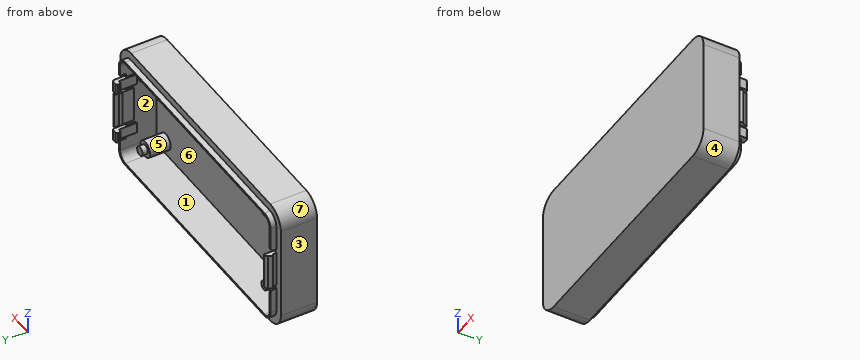
from build123d import *

# Parameters (mm, degrees)
EXTRUDE_2_DEPTH       = 10
EXTRUDE_4_DEPTH       = 1.6
SKETCH_7_W            = 0.5
SKETCH_7_H            = 10
EXTRUDE_8_DEPTH       = 2.8
SKETCH_8_R            = 0.7
EXTRUDE_9_DEPTH       = 10
FILLET_1_R            = 0.5
SKETCH_11_W           = 1
SKETCH_11_H           = 1.6
CUT_EXTRUDE_1_DEPTH   = 1.2
FILLET_2_R            = 1
SKETCH_13_W           = 0.5
SKETCH_13_H           = 10
EXTRUDE_10_DEPTH      = 2.8
CUT_EXTRUDE_START     = -8.5
CUT_EXTRUDE_2_DEPTH   = 8.5
SKETCH_13_2_W         = 0.5
SKETCH_13_2_H         = 10
EXTRUDE_11_DEPTH      = 2
EXTRUDE_12_DEPTH      = 1.6
EXTRUDE_12_DEPTH_BACK = 2
SKETCH_5_W            = 0.3
SKETCH_5_H            = 10
SKETCH_15_R           = 2.25
EXTRUDE_13_DEPTH      = 5.7
SKETCH_16_R           = 1.25
EXTRUDE_14_DEPTH      = 1.5
SKETCH_17_W           = 0.5
SKETCH_17_H           = 1
CUT_EXTRUDE_3_DEPTH   = 1.6
SKETCH_19_W           = 0.8
SKETCH_19_H           = 10
EXTRUDE_15_DEPTH      = 1.8
SKETCH_20_R           = 0.7
EXTRUDE_16_DEPTH      = 10
FILLET_4_R            = 0.5
SKETCH_21_W           = 0.5
SKETCH_21_H           = 3
EXTRUDE_17_DEPTH      = 1.9
SKETCH_22_W           = 3
SKETCH_22_H           = 6.3
EXTRUDE_23_DEPTH      = 0.5
FILLET_12_R           = 0.5
SKETCH_29_W           = 0.5
SKETCH_29_H           = 1
CUT_EXTRUDE_5_DEPTH   = 1.6
SKETCH_30_W           = 3
SKETCH_30_H           = 1.3
EXTRUDE_26_DEPTH      = 1
CHAMFER_7_SIZE        = 0.4


with BuildPart() as part:
    # case 2 → 凸台-拉伸2 (new body)
    with BuildSketch(Plane(origin=(0, 0, 0), x_dir=(1, 0, 0), z_dir=(0, 1, 0))):
        with BuildLine():
            Line((-34.042196447, 18), (30.957803553, 18))
            ThreePointArc((30.957803553, 18), (34.493337459, 16.535533906), (35.957803553, 13))
            Line((35.957803553, 13), (35.957803553, -13))
            ThreePointArc((35.957803553, -13), (34.493337459, -16.535533906), (30.957803553, -18))
            Line((30.957803553, -18), (-34.042196447, -18))
            ThreePointArc((-34.042196447, -18), (-37.577730353, -16.535533906), (-39.042196447, -13))
            Line((-39.042196447, -13), (-39.042196447, 13))
            ThreePointArc((-39.042196447, 13), (-37.577730353, 16.535533906), (-34.042196447, 18))
        make_face()
    extrude(amount=EXTRUDE_2_DEPTH)

    # 草图3 → 凸台-拉伸4 (add)
    with BuildSketch(Plane(origin=(0, 10, 0), x_dir=(1, 0, 0), z_dir=(0, 1, 0))):
        with BuildLine():
            Line((-36.942196447, 13), (-36.942196447, -13))
            ThreePointArc((-36.942196447, -13), (-36.092806113, -15.050609665), (-34.042196447, -15.9))
            Line((-34.042196447, -15.9), (30.957803553, -15.9))
            ThreePointArc((30.957803553, -15.9), (33.008413218, -15.050609665), (33.857803553, -13))
            Line((33.857803553, -13), (33.857803553, 13))
            ThreePointArc((33.857803553, 13), (33.008413218, 15.050609665), (30.957803553, 15.9))
            Line((30.957803553, 15.9), (-34.042196447, 15.9))
            ThreePointArc((-34.042196447, 15.9), (-36.092806113, 15.050609665), (-36.942196447, 13))
        make_face()
        with BuildLine():
            Line((-34.042196447, -15.4), (30.957803553, -15.4))
            ThreePointArc((30.957803553, -15.4), (32.654859828, -14.697056275), (33.357803553, -13))
            Line((33.357803553, -13), (33.357803553, 13))
            ThreePointArc((33.357803553, 13), (32.654859828, 14.697056275), (30.957803553, 15.4))
            Line((30.957803553, 15.4), (-34.042196447, 15.4))
            ThreePointArc((-34.042196447, 15.4), (-35.739252722, 14.697056275), (-36.442196447, 13))
            Line((-36.442196447, 13), (-36.442196447, -13))
            ThreePointArc((-36.442196447, -13), (-35.739252722, -14.697056275), (-34.042196447, -15.4))
        make_face(mode=Mode.SUBTRACT)
    extrude(amount=EXTRUDE_4_DEPTH)

    # 草图7 → 凸台-拉伸8 (add)
    with BuildSketch(Plane(origin=(0, 10, 0), x_dir=(1, 0, 0), z_dir=(0, 1, 0))):
        with Locations((-36.692196447, 0)):
            Rectangle(SKETCH_7_W, SKETCH_7_H)
    extrude(amount=EXTRUDE_8_DEPTH)

    # 草图8 → 凸台-拉伸9 (add)
    with BuildSketch(Plane.XY.offset(5)):
        with Locations((-36.692196447, 11.6)):
            Circle(SKETCH_8_R)
    extrude(amount=-EXTRUDE_9_DEPTH)

    # 圆角1
    fillet_1_edges = [part.edges().sort_by_distance(p)[0] for p in [
        (-36.942196447, 12.8, 0),
    ]]
    fillet(fillet_1_edges, radius=FILLET_1_R - 0.0001)  # a hair under: the kernel refuses the full size

    # 草图11 → 切除-拉伸1 (cut)
    with BuildSketch(Plane.ZY.offset(36.942196447)):
        with Locations((5.5, 10.8)):
            Rectangle(SKETCH_11_W, SKETCH_11_H)
        with Locations((-5.5, 10.8)):
            Rectangle(SKETCH_11_W, SKETCH_11_H)
    extrude(amount=-CUT_EXTRUDE_1_DEPTH, mode=Mode.SUBTRACT)

    # 圆角2
    fillet_2_edges = [part.edges().sort_by_distance(p)[0] for p in [
        (-36.692196447, 11.6, 6),
        (-36.692196447, 11.6, -6),
    ]]
    fillet(fillet_2_edges, radius=FILLET_2_R)

    # 草图13 → 凸台-拉伸10 (add)
    with BuildSketch(Plane(origin=(0, 10, 0), x_dir=(1, 0, 0), z_dir=(0, 1, 0))):
        with Locations((-36.192196447, 0)):
            Rectangle(SKETCH_13_W, SKETCH_13_H)
    extrude(amount=EXTRUDE_10_DEPTH)

    # 草图14 → 切除-拉伸2 (cut)
    with BuildSketch(Plane(origin=(0, 10, 0), x_dir=(1, 0, 0), z_dir=(0, 1, 0)).offset(CUT_EXTRUDE_START)):
        with BuildLine():
            Line((-34.042196447, -15.4), (30.957803553, -15.4))
            ThreePointArc((30.957803553, -15.4), (32.654859828, -14.697056275), (33.357803553, -13))
            Line((33.357803553, -13), (33.357803553, 13))
            ThreePointArc((33.357803553, 13), (32.654859828, 14.697056275), (30.957803553, 15.4))
            Line((30.957803553, 15.4), (-34.042196447, 15.4))
            ThreePointArc((-34.042196447, 15.4), (-35.739252722, 14.697056275), (-36.442196447, 13))
            Line((-36.442196447, 13), (-36.442196447, -13))
            ThreePointArc((-36.442196447, -13), (-35.739252722, -14.697056275), (-34.042196447, -15.4))
        make_face()
    extrude(amount=CUT_EXTRUDE_2_DEPTH, mode=Mode.SUBTRACT)

    # 草图13<2> → 凸台-拉伸11 (add)
    with BuildSketch(Plane(origin=(0, 10, 0), x_dir=(1, 0, 0), z_dir=(0, 1, 0))):
        with Locations((-36.192196447, 0)):
            Rectangle(SKETCH_13_2_W, SKETCH_13_2_H)
    extrude(amount=-EXTRUDE_11_DEPTH)

    # 草图5 → 凸台-拉伸12 (add, two sides: drawn at the far end of the back side and taken through both)
    with BuildSketch(Plane(origin=(0, 10, 0), x_dir=(1, 0, 0), z_dir=(0, 1, 0)).offset(-EXTRUDE_12_DEPTH_BACK)):
        with Locations((33.207803553, 0)):
            Rectangle(SKETCH_5_W, SKETCH_5_H)
    extrude(amount=EXTRUDE_12_DEPTH + EXTRUDE_12_DEPTH_BACK)

    # 草图15 → 凸台-拉伸13 (add)
    with BuildSketch(Plane(origin=(0, 1.5, 0), x_dir=(1, 0, 0), z_dir=(0, 1, 0))):
        with Locations(Location((29.060337171, -11.529492838, 0), (0, 0, 270))):
            Circle(SKETCH_15_R)
        with Locations(Location((-28.939662829, -11.529492838, 0), (0, 0, 270))):
            Circle(SKETCH_15_R)
        with Locations(Location((29.060337171, 11.470507162, 0), (0, 0, 270))):
            Circle(SKETCH_15_R)
        with Locations(Location((-28.939662829, 11.470507162, 0), (0, 0, 270))):
            Circle(SKETCH_15_R)
    extrude(amount=EXTRUDE_13_DEPTH)

    # 草图16 → 凸台-拉伸14 (add)
    with BuildSketch(Plane(origin=(0, 7.2, 0), x_dir=(1, 0, 0), z_dir=(0, 1, 0))):
        with Locations(Location((29.060337171, -11.529492838, 0), (0, 0, 270))):
            Circle(SKETCH_16_R)
        with Locations(Location((29.060337171, 11.470507162, 0), (0, 0, 270))):
            Circle(SKETCH_16_R)
        with Locations(Location((-28.939662829, -11.529492838, 0), (0, 0, 270))):
            Circle(SKETCH_16_R)
        with Locations(Location((-28.939662829, 11.470507162, 0), (0, 0, 270))):
            Circle(SKETCH_16_R)
    extrude(amount=EXTRUDE_14_DEPTH)

    # 草图17 → 切除-拉伸3 (cut)
    with BuildSketch(Plane(origin=(0, 11.6, 0), x_dir=(1, 0, 0), z_dir=(0, 1, 0))):
        with Locations((33.607803553, -5.5)):
            Rectangle(SKETCH_17_W, SKETCH_17_H)
        with Locations((33.607803553, 5.5)):
            Rectangle(SKETCH_17_W, SKETCH_17_H)
    extrude(amount=-CUT_EXTRUDE_3_DEPTH, mode=Mode.SUBTRACT)

    # 草图19 → 凸台-拉伸15 (add)
    with BuildSketch(Plane(origin=(0, 11.6, 0), x_dir=(1, 0, 0), z_dir=(0, 1, 0))):
        with Locations((33.457803553, 0)):
            Rectangle(SKETCH_19_W, SKETCH_19_H)
    extrude(amount=EXTRUDE_15_DEPTH)

    # 草图20 → 凸台-拉伸16 (add)
    with BuildSketch(Plane(origin=(0, 0, -5), x_dir=(-1, 0, 0), z_dir=(0, 0, -1))):
        with Locations((-33.607803553, 11.6)):
            Circle(SKETCH_20_R)
    extrude(amount=-EXTRUDE_16_DEPTH)

    # 圆角4
    fillet_4_edges = [part.edges().sort_by_distance(p)[0] for p in [
        (33.857803553, 13.4, 0),
    ]]
    fillet(fillet_4_edges, radius=FILLET_4_R)

    # 草图21 → 凸台-拉伸17 (add)
    with BuildSketch(Plane(origin=(0, 11.6, 0), x_dir=(1, 0, 0), z_dir=(0, 1, 0))):
        with Locations((33.607803553, -7.5)):
            Rectangle(SKETCH_21_W, SKETCH_21_H)
        with Locations((33.607803553, 7.5)):
            Rectangle(SKETCH_21_W, SKETCH_21_H)
    extrude(amount=EXTRUDE_17_DEPTH)

    # 草图22 → 凸台-拉伸23 (add)
    with BuildSketch(Plane.ZY.offset(-33.357803553)):
        with Locations((-7.5, 10.35)):
            Rectangle(SKETCH_22_W, SKETCH_22_H)
        with Locations((7.5, 10.35)):
            Rectangle(SKETCH_22_W, SKETCH_22_H)
    extrude(amount=EXTRUDE_23_DEPTH)

    # 圆角12
    fillet_12_edges = [part.edges().sort_by_distance(p)[0] for p in [
        (33.857803553, 13.5, 7.5),
        (33.857803553, 13.5, -7.5),
    ]]
    fillet(fillet_12_edges, radius=FILLET_12_R)

    # 草图29 → 切除-拉伸5 (cut)
    with BuildSketch(Plane(origin=(0, 11.6, 0), x_dir=(1, 0, 0), z_dir=(0, 1, 0))):
        with Locations((33.607803553, -9.5)):
            Rectangle(SKETCH_29_W, SKETCH_29_H)
        with Locations((33.607803553, 9.5)):
            Rectangle(SKETCH_29_W, SKETCH_29_H)
    extrude(amount=-CUT_EXTRUDE_5_DEPTH, mode=Mode.SUBTRACT)

    # 草图30 → 凸台-拉伸26 (add)
    with BuildSketch(Plane.ZY.offset(-32.857803553)):
        with Locations((7.5, 12.85)):
            Rectangle(SKETCH_30_W, SKETCH_30_H)
        with Locations((-7.5, 12.85)):
            Rectangle(SKETCH_30_W, SKETCH_30_H)
    extrude(amount=EXTRUDE_26_DEPTH)

    # 倒角7
    chamfer_7_edges = [part.edges().sort_by_distance(p)[0] for p in [
        (31.857803553, 12.2, 7.5),
        (31.857803553, 13.5, 7.5),
        (31.857803553, 12.2, -7.5),
        (31.857803553, 13.5, -7.5),
    ]]
    chamfer(chamfer_7_edges, length=CHAMFER_7_SIZE)


solid = part.part
For this review, take the finished solid that the model builds, in its own axes (mm). Face numbers are marked on the shaded views. A direction names the side the tool comes from. Round coordinates to 2 decimals unless told otherwise and drop trailing zeros. Write each loop counter-clockwise with the first axis right and the second up, starting at its lowest first coordinate (ties: lowest second). Pieces come first, ordered by that corner, then holes. Notation, with made-up numbers: M -25.5,37 L -20.5,37 A33 ccw -20.5,69 Z; hole C -37,78.25 d7. An arc over 180 degrees is marked long. Write item = value, one per line. Start each with the question number.
(1) We need section B-B (z = 0). Give the boundary of the cut face in (x, y), then the cut area to 3 significant figures.
(2) We need section D-D (z = 11). Give the boundary of the cut face in (x, y).
(3) For the marked faces 1, 2 and 3, list the 3-axis set-ups (+Z, -Z, +X, -X, +Y, -Y) from which the entire face can be reached by the end or side of a thin tool; tool diameter is ignored.
(4) We need section A-A (y = 3.75). Give the boundary of the cut face in (x, z), then the cut area to 3 significant figures.
(5) Clearance check with flat-ended pins moving along their axes: pin 1 Ø0.6 at (y, z) = (13, 7) entering from -X; pin 2 Ø0.8 at (x, z) = (-29, -11.5) entering from +Y; pin 3 Ø10 at (x, z) = (10.5, -10.5) entering from -Y; pin 4 Ø3.5 at (y, z) = (12, 7.5) entering from +X. State where each tip first meets the part, or that it passes through.
(6) For line 1 along X through (y, z) = (11.25, -7); line 2 along Z through (x, y) = (14, 10.5); line 3 along X through (y, z) = (10.25, -2.5), list the stretches that pass through material, from the lowest coordinate up.
(7) We need section C-C (x = -25). Give the boundary of the cut face in (y, z), then the cut area to 3 significant figures.
(8) The part is to be moulded in two halves that separate along Z. For the marked faces 4, 5, 6 and 7, say which applies: +Z half, -Z half, draft (parallel to the pull), parting line (faces both ways), or undercut.
Results found:
q1.outline = M -39.04,0 L 35.96,0 L 35.96,10 L 33.86,10 L 33.86,10.95 A0.7 ccw 33.86,12.25 L 33.86,12.9 A0.5 ccw 33.36,13.4 L 33.06,13.4 L 33.06,12.03 A0.7 ccw 33.06,11.17 L 33.06,8 L 33.36,8 L 33.36,1.5 L -36.44,1.5 L -36.44,8 L -35.94,8 L -35.94,12.8 L -36.44,12.8 A0.5 ccw -36.94,12.3 L -36.94,12.25 A0.7 ccw -36.94,10.95 L -36.94,10 L -39.04,10 Z
q1.area = 165 mm²
q2.outline = M -39.04,0 L 35.96,0 L 35.96,10 L 33.86,10 L 33.86,11.6 L 33.36,11.6 L 33.36,1.5 L 31.25,1.5 L 31.25,7.2 L 30.19,7.2 L 30.19,8.7 L 27.93,8.7 L 27.93,7.2 L 26.87,7.2 L 26.87,1.5 L -26.75,1.5 L -26.75,7.2 L -27.81,7.2 L -27.81,8.7 L -30.07,8.7 L -30.07,7.2 L -31.13,7.2 L -31.13,1.5 L -36.44,1.5 L -36.44,11.6 L -36.94,11.6 L -36.94,10 L -39.04,10 Z
q3.face_1 = +Y
q3.face_2 = none
q3.face_3 = +Z, -Z, -X, +Y, -Y
q4.outline = M -39.04,-13 A5 ccw -34.04,-18 L 30.96,-18 A5 ccw 35.96,-13 L 35.96,13 A5 ccw 30.96,18 L -34.04,18 A5 ccw -39.04,13 Z; C -28.94,-11.47 d4.5; C -28.94,11.53 d4.5; C 29.06,-11.47 d4.5; C 29.06,11.53 d4.5; hole M -36.44,-13 A2.4 ccw -34.04,-15.4 L 30.96,-15.4 A2.4 ccw 33.36,-13 L 33.36,13 A2.4 ccw 30.96,15.4 L -34.04,15.4 A2.4 ccw -36.44,13 Z
q4.area = 597 mm²
q5.pin_1 = 31.86
q5.pin_2 = 8.7
q5.pin_3 = 0
q5.pin_4 = 33.86
q6.line_1 = -36.94 to -36.44, 32.86 to 33.86
q6.line_2 = -15.9 to -15.4, 15.4 to 15.9
q6.line_3 = -36.94 to -35.94, 33.06 to 33.86
q7.outline = M 0,-18 L 10,-18 L 10,-15.9 L 11.6,-15.9 L 11.6,-15.4 L 1.5,-15.4 L 1.5,15.4 L 11.6,15.4 L 11.6,15.9 L 10,15.9 L 10,18 L 0,18 Z
q7.area = 99.8 mm²
q8.face_4 = -Z half
q8.face_5 = undercut
q8.face_6 = undercut
q8.face_7 = +Z half
